```python
from build123d import *

# Parameters (mm, degrees)
F0_R      = 1.525
F0_R_2    = 13
F1_DEPTH  = 7.6
F0_R_3    = 6.5
F2_DEPTH  = 6
F3_DEPTH  = 3
F4_DEPTH  = 6
F5_DEPTH  = 2
F6_SIZE2  = 5
F6_SIZE   = 4
F7_SIZE2  = 1.5
F7_SIZE   = 4
F8_R      = 1.5
F11_DEPTH = 45
F12_DEPTH = 10
F9_R      = 1.5
F13_DEPTH = 10
F14_DEPTH = 10
F10_R     = 1.5
F15_DEPTH = 15
F16_DEPTH = 10


with BuildPart() as f1:
    # F0 (on Top) → F1 (new body)
    with BuildSketch(Plane.XY):
        with BuildLine():
            Line((11.4654492345, 28.1041493633), (11.4654492345, 17.6041493633))
            Line((11.4654492345, 17.6041493633), (21.5054492345, 17.6041493633))
            Line((21.5054492345, 17.6041493633), (21.5054492345, 28.1041493633))
            Line((21.5054492345, 28.1041493633), (11.5113214177, 49.4730095995))
            Line((11.5113214177, 49.4730095995), (5.4613214177, 49.4730095995))
            Line((5.4613214177, 49.4730095995), (-66.2845185672, 19.8239773236))
            Line((-66.2845185672, 19.8239773236), (-66.2845185672, 17.5239773236))
            Line((-66.2845185672, 17.5239773236), (-56.2845185672, 17.5239773236))
            Line((-56.2845185672, 17.5239773236), (-56.2845185672, 8.8239773236))
            Line((-56.2845185672, 8.8239773236), (-66.2845185672, 8.8239773236))
            Line((-66.2845185672, 8.8239773236), (-76.0307126449, -46.6298285987))
            Line((-76.0307126449, -46.6298285987), (-71.4345185672, -51.2260226764))
            Line((-71.4345185672, -51.2260226764), (-61.2180819327, -51.1889110274))
            Line((-61.2180819327, -51.1889110274), (-55.7966974161, -46.606532264))
            Line((-55.7966974161, -46.606532264), (-51.9234810694, -51.1889110274))
            Line((-51.9234810694, -51.1889110274), (-48.9812307256, -51.1833146176))
            ThreePointArc((-48.9812307256, -51.1833146176), (-55.8366672394, -42.5867224617), (-57.6113446632, -31.7355047176))
            ThreePointArc((-57.6113446632, -31.7355047176), (-62.7216685586, -26.760327644), (-55.8293902254, -24.9261257448))
            ThreePointArc((-55.8293902254, -24.9261257448), (-49.3810695109, -16.6521794806), (-39.8099914805, -12.3587551881))
            ThreePointArc((-39.8099914805, -12.3587551881), (-27.7993054872, -13.6020861151), (-18.3026540226, -21.0597037496))
            Line((-18.3026540226, -21.0597037496), (-5.0345507655, 8.4941493633))
            Line((-5.0345507655, 8.4941493633), (-5.0345507655, 17.6041493633))
            Line((-5.0345507655, 17.6041493633), (2.7154492345, 17.6041493633))
            Line((2.7154492345, 17.6041493633), (2.7154492345, 28.1041493633))
            Line((2.7154492345, 28.1041493633), (11.4654492345, 28.1041493633))
        make_face()
        with BuildLine():
            Line((-36.8574590489, -11.8271979792), (-39.8099914805, -12.3587551881))
            Line((-39.8099914805, -12.3587551881), (-42.7625236411, -12.8903123481))
            Line((-42.7625236411, -12.8903123481), (-47.1873519708, 11.6873792538))
            Line((-47.1873519708, 11.6873792538), (-47.1921668449, 11.7141234529))
            ThreePointArc((-47.1921668449, 11.7141234529), (-44.7687897478, 15.1848711151), (-41.2871022526, 12.7772378218))
            Line((-41.2871022526, 12.7772378218), (-41.2822873786, 12.7504936227))
            Line((-41.2822873786, 12.7504936227), (-36.8574590489, -11.8271979792))
        make_face(mode=Mode.SUBTRACT)
        with Locations((-31.119161509, 13.4325037545)):
            Circle(F0_R, mode=Mode.SUBTRACT)
        with Locations((6.6226837225, 38.0824916065)):
            Circle(F0_R, mode=Mode.SUBTRACT)
        with BuildLine():
            ThreePointArc((-48.9812307256, -51.1833146176), (-20.7176395084, -49.2839158598), (-18.3026540226, -21.0597037496))
            ThreePointArc((-18.3026540226, -21.0597037496), (-27.7993054872, -13.6020861151), (-39.8099914805, -12.3587551881))
            ThreePointArc((-39.8099914805, -12.3587551881), (-49.3810695109, -16.6521794806), (-55.8293902254, -24.9261257448))
            ThreePointArc((-55.8293902254, -24.9261257448), (-54.9601088644, -26.2468514875), (-54.6552348922, -27.7983083618))
            ThreePointArc((-54.6552348922, -27.7983083618), (-55.4765194472, -30.2600201708), (-57.6113446632, -31.7355047176))
            ThreePointArc((-57.6113446632, -31.7355047176), (-55.8366672394, -42.5867224617), (-48.9812307256, -51.1833146176))
        make_face()
        Polygon((-50.1124866335, -41.8020018535), (-46.2392702868, -46.3843806169), (-48.33952722, -48.1596047758), (-52.2127435668, -43.5772260124), align=None, mode=Mode.SUBTRACT)
        with Locations((-35.9562017577, -33.7646143106)):
            Circle(F0_R_2, mode=Mode.SUBTRACT)
        Polygon((-41.7437057042, -18.5493325824), (-42.2309664567, -15.8428446443), (-36.3259018644, -14.7797302754), (-35.838641112, -17.4862182135), align=None, mode=Mode.SUBTRACT)
        Polygon((-22.0480286327, -41.9629163019), (-19.7605397552, -36.416079849), (-17.2182397143, -37.4645122512), (-19.5057285918, -43.0113487041), align=None, mode=Mode.SUBTRACT)
    extrude(amount=F1_DEPTH)

    # F0 (on Top) → F2 (join)
    with BuildSketch(Plane.XY):
        with BuildLine():
            ThreePointArc((-48.9812307256, -51.1833146176), (-20.7176395084, -49.2839158598), (-18.3026540226, -21.0597037496))
            ThreePointArc((-18.3026540226, -21.0597037496), (-27.7993054872, -13.6020861151), (-39.8099914805, -12.3587551881))
            ThreePointArc((-39.8099914805, -12.3587551881), (-49.3810695109, -16.6521794806), (-55.8293902254, -24.9261257448))
            ThreePointArc((-55.8293902254, -24.9261257448), (-54.9601088644, -26.2468514875), (-54.6552348922, -27.7983083618))
            ThreePointArc((-54.6552348922, -27.7983083618), (-55.4765194472, -30.2600201708), (-57.6113446632, -31.7355047176))
            ThreePointArc((-57.6113446632, -31.7355047176), (-55.8366672394, -42.5867224617), (-48.9812307256, -51.1833146176))
        make_face()
        Polygon((-50.1124866335, -41.8020018535), (-46.2392702868, -46.3843806169), (-48.33952722, -48.1596047758), (-52.2127435668, -43.5772260124), align=None, mode=Mode.SUBTRACT)
        with Locations((-35.9562017577, -33.7646143106)):
            Circle(F0_R_2, mode=Mode.SUBTRACT)
        Polygon((-41.7437057042, -18.5493325824), (-42.2309664567, -15.8428446443), (-36.3259018644, -14.7797302754), (-35.838641112, -17.4862182135), align=None, mode=Mode.SUBTRACT)
        Polygon((-22.0480286327, -41.9629163019), (-19.7605397552, -36.416079849), (-17.2182397143, -37.4645122512), (-19.5057285918, -43.0113487041), align=None, mode=Mode.SUBTRACT)
        with Locations((-35.9562017577, -33.7646143106)):
            Circle(F0_R_2)
        with Locations((-35.9562017577, -33.7646143106)):
            Circle(F0_R_3, mode=Mode.SUBTRACT)
    extrude(amount=-F2_DEPTH)

    # F0 (on Top) → F3 (cut)
    with BuildSketch(Plane.XY):
        with Locations((-35.9562017577, -33.7646143106)):
            Circle(F0_R_2)
        with Locations((-35.9562017577, -33.7646143106)):
            Circle(F0_R_3, mode=Mode.SUBTRACT)
    extrude(amount=-F3_DEPTH, mode=Mode.SUBTRACT)

    # F0 (on Top) → F4 (join)
    with BuildSketch(Plane.XY):
        Polygon((-48.33952722, -48.1596047758), (-46.2392702868, -46.3843806169), (-50.1124866335, -41.8020018535), (-52.2127435668, -43.5772260124), align=None)
        Polygon((-36.3259018644, -14.7797302754), (-42.2309664567, -15.8428446443), (-41.7437057042, -18.5493325824), (-35.838641112, -17.4862182135), align=None)
        Polygon((-17.2182397143, -37.4645122512), (-19.7605397552, -36.416079849), (-22.0480286327, -41.9629163019), (-19.5057285918, -43.0113487041), align=None)
    extrude(amount=-F4_DEPTH)

    # F0 (on Top) → F5 (cut)
    with BuildSketch(Plane.XY):
        Polygon((-36.3259018644, -14.7797302754), (-42.2309664567, -15.8428446443), (-41.7437057042, -18.5493325824), (-35.838641112, -17.4862182135), align=None)
        Polygon((-17.2182397143, -37.4645122512), (-19.7605397552, -36.416079849), (-22.0480286327, -41.9629163019), (-19.5057285918, -43.0113487041), align=None)
        Polygon((-48.33952722, -48.1596047758), (-46.2392702868, -46.3843806169), (-50.1124866335, -41.8020018535), (-52.2127435668, -43.5772260124), align=None)
    extrude(amount=-F5_DEPTH, mode=Mode.SUBTRACT)

    # F6
    f6_edges = [f1.edges().sort_by_distance(p)[0] for p in [
        (-44.76879, 15.184871, 7.6),
        (-39.072281, 0.47502, 7.6),
        (-44.977345, -0.588094, 7.6),
    ]]
    f6_side = f1.faces().sort_by_distance((-32.346153, -0.818971, 7.6))[0]
    chamfer(f6_edges, length=F6_SIZE, length2=F6_SIZE2, reference=f6_side)

    # F7
    f7_edges = [f1.edges().sort_by_distance(p)[0] for p in [
        (-39.072281, 0.47502, 0),
        (-44.977345, -0.588094, 0),
        (-44.76879, 15.184871, 0),
    ]]
    f7_side = f1.faces().sort_by_distance((-31.55219, 6.99064, 0))[0]
    chamfer(f7_edges, length=F7_SIZE, length2=F7_SIZE2, reference=f7_side)

    # F8 (on face) → F11 (cut)
    with BuildSketch(Plane(origin=(1.4368780264, -7.9811333617, 0), x_dir=(0.984177432, 0.1771857282, 0), z_dir=(0.1771857282, -0.984177432, 0))):
        with Locations((-41.3698900842, 2)):
            Circle(F8_R)
    extrude(amount=-F11_DEPTH, mode=Mode.SUBTRACT)

    # F8 (on face) → F12 (cut)
    with BuildSketch(Plane(origin=(1.4368780264, -7.9811333617, 0), x_dir=(0.984177432, 0.1771857282, 0), z_dir=(0.1771857282, -0.984177432, 0))):
        with Locations((-41.3698900842, 2)):
            Circle(F8_R)
    extrude(amount=F12_DEPTH, mode=Mode.SUBTRACT)

    # F9 (on face) → F13 (cut)
    with BuildSketch(Plane(origin=(-1.5110668178, 0.6231567432, 0), x_dir=(-0.3812481463, -0.9244727422, 0), z_dir=(-0.9244727422, 0.3812481463, 0))):
        with Locations((44.199342347, 2)):
            Circle(F9_R)
    extrude(amount=-F13_DEPTH, mode=Mode.SUBTRACT)

    # F9 (on face) → F14 (cut)
    with BuildSketch(Plane(origin=(-1.5110668178, 0.6231567432, 0), x_dir=(-0.3812481463, -0.9244727422, 0), z_dir=(-0.9244727422, 0.3812481463, 0))):
        with Locations((44.199342347, 2)):
            Circle(F9_R)
    extrude(amount=F14_DEPTH, mode=Mode.SUBTRACT)

    # F10 (on face) → F15 (cut)
    with BuildSketch(Plane(origin=(-51.939047377, -43.9010343142, 0), x_dir=(-0.6455360578, 0.7637297939, 0), z_dir=(0.7637297939, 0.6455360578, 0))):
        with Locations((-2.576017193, 2)):
            Circle(F10_R)
    extrude(amount=-F15_DEPTH, mode=Mode.SUBTRACT)

    # F10 (on face) → F16 (cut)
    with BuildSketch(Plane(origin=(-51.939047377, -43.9010343142, 0), x_dir=(-0.6455360578, 0.7637297939, 0), z_dir=(0.7637297939, 0.6455360578, 0))):
        with Locations((-2.576017193, 2)):
            Circle(F10_R)
    extrude(amount=F16_DEPTH, mode=Mode.SUBTRACT)


solid = f1.part
```
Check sheet for the modelled part. Datum: model origin and axes. Units: mm. A direction names the side the tool comes from. Round coordinates to 2 decimals unless told otherwise and drop trailing zeros. Order: outer loops, then holes, each group sorted by start corner. A loop starts at its lowest first (then second) coordinate and runs counter-clockwise, first axis right, second up. Notation, with made-up numbers: (79.25, 41) -> (120.25, 41) arc R17 ccw to (120.25, 47) -> close; hole circle Ø9 at (64.25, 41). An arc over 180 degrees is marked (long way). Use CSV: the item, a comma, the result in double quotes.
(1) Cross-section at C-C (z = -4.75). Record the boundary of the cut face in (x, y), and give its area (3 significant figures).
Worked out:
outline,"(-57.61, -31.74) arc R21.75 ccw (long way) to (-55.83, -24.93) arc R4.1 cw to start; hole circle Ø13 at (-35.96, -33.76)"
area,"1,340 mm²"
(2) Tool access check on faces 5 (the face through (-56.285, 13, 4)), 6 (the face through (-11.76, -6.49, 3.75)), 7 (the face through (-46.365, 15.717, 1.094)), 8 (the face through (-66.285, 19, 4)). Record the directions out of +Z, -Z, +X, -X, +Y, -Y that give a thin tool (end or side, any length) a straight path to the whole face; none if there is none.
Worked out:
face 5,"+Z, -Z, -X"
face 6,"+Z, -Z, +X"
face 7,"-Z"
face 8,"+Z, -Z, -X, +Y"
(3) Cross-section at D-D (x = 1). Record the boundary of the cut face in (y, z), and give its area (3 significant figures).
Worked out:
outline,"(17.6, 0) -> (47.63, 0) -> (47.63, 7.6) -> (17.6, 7.6) -> close"
area,"228 mm²"
(4) Depth check by flat-ended pin: pin 1 (4 mm diameter, centred on x = -11.5, y = 1.5, fed in from -Z); pin 2 (2.5 mm diameter, centred on y = 13, z = 2, fed in from -X); pin 3 (4 mm diameter, centred on y = 23.5, z = 5, fed in from -X). Enter the tip coordinate at first touch or a pass-through.
Worked out:
pin 1,"z = 0"
pin 2,"x = -56.28"
pin 3,"x = -62.23"
(5) Cross-section at B-B (y = 21.5). Count the separate pieces of the cut face and the enclosed holes in it, and give its area (3 significant figures).
Worked out:
separate pieces,"2"
enclosed holes,"1"
area,"563 mm²"
(6) Cross-section at A-A (y = -2). Record the boundary of the cut face in (x, z).
Worked out:
outline,"(-68.19, 0) -> (-48.79, 0) -> (-44.72, 1.5) -> (-44.72, 2.6) -> (-48.79, 7.6) -> (-68.19, 7.6) -> close; (-38.63, 1.5) -> (-34.56, 0) -> (-9.75, 0) -> (-9.75, 7.6) -> (-34.56, 7.6) -> (-38.63, 2.6) -> close"
(7) Draft check along Y on faces 1 (the face through (-61, 17.524, 4)), 2 (the face through (-1, 17.604, 4)), 3 (the face through (-28, 11, 0)), 4 (the face through (-29.909, 34.856, 3.747)). Enter one of: pulls with the +Y half, pulls with the -Y half, needs draft (parallel to the pull), parting line crosses it, or undercut.
Worked out:
face 1,"undercut"
face 2,"pulls with the -Y half"
face 3,"needs draft"
face 4,"pulls with the +Y half"
(8) Material ranges on line 1 along Y through (x, z) = (-62.5, 4); line 2 along X through (y, z) = (19.5, 4.75); line 3 along Y through (x, z) = (-59, 4), recorded low to high. Write a range as from..to.
Worked out:
line 1,"-51.19..-29.47, -26.13..8.82, 17.52..21.39"
line 2,"-66.28..2.72, 11.47..21.51"
line 3,"-49.31..-31.89, -23.71..8.82, 17.52..22.83"
